Can you work these out from the model? Positions are in its coordinate system, mm. A direction names the side the tool comes from. Round coordinates to 2 decimals unless told otherwise and drop trailing zeros. Loops run counter-clockwise (first coordinate to the right, second up) from the corner with the lowest first, then second, coordinate; pieces in that order, holes last. Notation, with made-up numbers: (-19.5, -25) -> (0.5, -25) arc R35 cw to (0.5, 9) -> close; hole circle Ø4 at (85.5, -30.5). An arc over 180 degrees is marked (long way). Write item = value, one per line.
from build123d import *

# Parameters (mm, degrees)
SKETCH1_W           = 14
SKETCH1_H           = 16
BOSS_EXTRUDE1_DEPTH = 20
CUT_EXTRUDE1_DEPTH  = 5
CHAMFER1_SIZE       = 2
CHAMFER2_SIZE       = 1
SKETCH4_R           = 5
CUT_EXTRUDE2_DEPTH  = 12


with BuildPart() as part:
    # Sketch1 → Boss-Extrude1 (new body)
    with BuildSketch(Plane(origin=(0, 0, 0), x_dir=(1, 0, 0), z_dir=(0, 1, 0))):
        with Locations((7, 8)):
            Rectangle(SKETCH1_W, SKETCH1_H)
    extrude(amount=-BOSS_EXTRUDE1_DEPTH)

    # Sketch2 → Cut-Extrude1 (cut)
    with BuildSketch(Plane(origin=(0, 0, 0), x_dir=(1, 0, 0), z_dir=(0, 1, 0))):
        Polygon((3, 6), (0, 6), (0, 5), (8, 5), (8, 0), (14, 0), (14, 6), (10.5, 6), (10.5, 16), (10, 16), (10, 6), (7, 6), (7, 16), (6.5, 16), (6.5, 6), (3.5, 6), (3.5, 16), (3, 16), align=None)
    extrude(amount=-CUT_EXTRUDE1_DEPTH, mode=Mode.SUBTRACT)

    # Chamfer1
    chamfer1_edges = [part.edges().sort_by_distance(p)[0] for p in [
        (8.5, 0, -16),
        (5, 0, -16),
        (1.5, 0, -16),
        (12.25, 0, -16),
    ]]
    chamfer(chamfer1_edges, length=CHAMFER1_SIZE)

    # Chamfer2
    chamfer2_edges = [part.edges().sort_by_distance(p)[0] for p in [
        (8, -2.5, 0),
        (4, 0, 0),
        (0, -11, -16),
        (14, -11, -16),
        (14, -12.5, 0),
        (0, -10, 0),
    ]]
    chamfer(chamfer2_edges, length=CHAMFER2_SIZE)

    # Sketch4 → Cut-Extrude2 (cut)
    with BuildSketch(Plane.XZ.offset(20)):
        with Locations(Location((7, -8, 0), (0, 0, 270))):
            Circle(SKETCH4_R)
    extrude(amount=-CUT_EXTRUDE2_DEPTH, mode=Mode.SUBTRACT)


solid = part.part
1. I'm going to push flat-ended pins straight in: pin 1 (6 mm diameter, centred on x = 7, z = -8, fed in from -Y); pin 2 (2 mm diameter, centred on y = -3, z = -3.5, fed in from +X); pin 3 (1.8 mm diameter, centred on x = 11.5, y = -3.5, fed in from +Z). Where does each tip first touch, or does it pass through?
Entries:
pin_1 = -8
pin_2 = 8
pin_3 = -6
2. Suppose I cut it at D-D, the plane z = -8. List the corners of the cut face in (x, y) for me.
Entries:
outline = (0, -20) -> (2, -20) -> (2, -8) -> (12, -8) -> (12, -20) -> (14, -20) -> (14, 0) -> (10.5, 0) -> (10.5, -5) -> (10, -5) -> (10, 0) -> (7, 0) -> (7, -5) -> (6.5, -5) -> (6.5, 0) -> (3.5, 0) -> (3.5, -5) -> (3, -5) -> (3, 0) -> (0, 0) -> close
3. Suppose I cut it at B-B, the plane x = 1.75. List the corners of the cut face in (y, z) for me, and give its area (4 significant figures).
Entries:
outline = (-20, -16) -> (-2, -16) -> (0, -14) -> (0, -6) -> (-5, -6) -> (-5, -5) -> (0, -5) -> (0, -1) -> (-1, 0) -> (-20, 0) -> close
area = 312.5 mm²
4. Suppose I cut it at C-C, the plane y = -3.75. List the corners of the cut face in (x, z) for me, and give its area (3 significant figures).
Entries:
outline = (0, -15) -> (1, -16) -> (3, -16) -> (3, -6) -> (0, -6) -> close; (0, -5) -> (8, -5) -> (8, -1) -> (7, 0) -> (1, 0) -> (0, -1) -> close; (3.5, -16) -> (6.5, -16) -> (6.5, -6) -> (3.5, -6) -> close; (7, -16) -> (10, -16) -> (10, -6) -> (7, -6) -> close; (10.5, -16) -> (13, -16) -> (14, -15) -> (14, -6) -> (10.5, -6) -> close
area = 163 mm²
5. We'd pull the mould along Z, two halves only. Please class faces 1 (the flat face through (7.5, -2.5, -0.5)), 2 (the flat face through (10, -2, -11)), 3 (the flat face through (2, -2, -6)): released by +Z, released by -Z, zero draft, split by the parting line, or undercut.
Entries:
face_1 = released by +Z
face_2 = zero draft
face_3 = undercut
6. For faces 4 (the flat face through (8, -2, -3)), 5 (the flat face through (7, -11, -16)), 6 (the flat face through (4, -2, -5)), 7 (the flat face through (6.5, -2, -11)), which set-ups out of +Z, -Z, +X, -X, +Y, -Y let a thin tool reach every point of the face, with its end or its side?
Entries:
face_4 = +Z, +X, +Y
face_5 = -Z, +X, -X, +Y, -Y
face_6 = +X, -X, +Y
face_7 = -Z, +Y
7. Suppose I cut it at A-A, the plane y = -10. List the corners of the cut face in (x, z) for me.
Entries:
outline = (0, -15) -> (1, -16) -> (13, -16) -> (14, -15) -> (14, -1) -> (13, 0) -> (1, 0) -> (0, -1) -> close; hole circle Ø10 at (7, -8)
8. I need wall thicknesses on line 1 (X direction, y = -0.75, z = -14.5); line 2 (X direction, y = -10.25, z = -8); line 3 (Y direction, x = 9, z = -1.5). Which ranges of each line are inside material? Lowest first, please. Write a range as [from, to].
Entries:
line_1 = [0, 3], [3.5, 6.5], [7, 10], [10.5, 14]
line_2 = [0, 2], [12, 14]
line_3 = [-20, -5]
